Design review of the part built by this model. Coordinates are the model's own, in mm. Face numbers are marked on the shaded views. A direction names the side the tool comes from. Coordinates: 2 decimals unless noted, no trailing zeros. Order: outer loops, then holes, each group sorted by start corner. A loop starts at its lowest first (then second) coordinate and runs counter-clockwise, first axis right, second up. Notation, with made-up numbers: M -2,57 L 21,57 A12 cw 21,65 Z; hole C -18,23.5 d9. An arc over 180 degrees is marked long. Use CSV: the item, a comma, the result in double quotes.
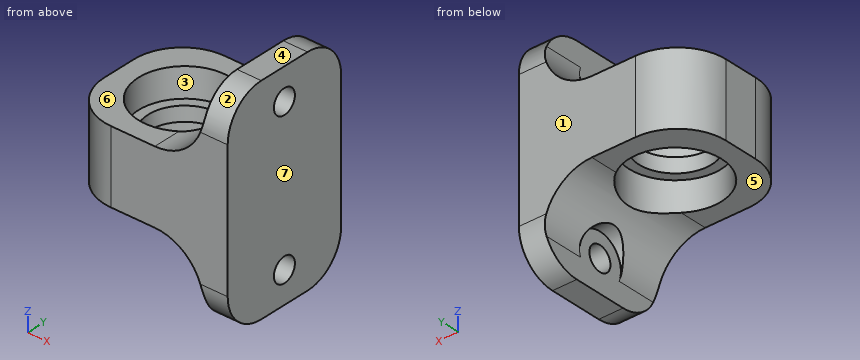
Autodesk Inventor part; units mm, degrees
ref_plane "YZ Plane" through (0, 0, 0) normal (1, 0, 0) x (0, 1, 0)
ref_plane "XZ Plane" through (0, 0, 0) normal (0, 1, 0) x (-1, 0, 0)
ref_plane "XY Plane" through (0, 0, 0) normal (0, 0, 1) x (1, 0, 0)
sketch "Szkic1" plane through (0, 0, 0) normal (0, 0, 1) x (1, 0, 0)
  line L0 (-15.5705, 13.388) -> (18.4295, 13.388)
  line L1 (18.4295, 13.388) -> (18.4295, -13.612)
  line L2 (18.4295, -13.612) -> (-15.5705, -13.612)
  line L3 (-15.5705, -13.612) -> (-15.5705, 13.388)
  circle A0 centre (-2.0705, -0.112) radius 9.5
  point P0 (0, 0)
  dimension "d0" = 27
  dimension "d1" = 34
  dimension "d2" = 20.5
  dimension "d3" = 13.5
  dimension "d4" = 19
extrude "Wyciągnięcie proste1" add sketch "Szkic1" along normal blind 15 contours L0 L1 L2 L3 | A0
extrude "Wyciągnięcie proste2" cut sketch "Szkic1" along normal blind 6 contours A0
sketch "Szkic2" plane through (0, 0, 15) normal (0, 0, 1) x (1, 0, 0)
  circle A0 centre (-2.0705, -0.112) radius 9.5
  line L0 (18.4295, 13.388) -> (-15.5705, 13.388)
  line L1 (-15.5705, 13.388) -> (-15.5705, -13.612)
  line L2 (-15.5705, -13.612) -> (18.4295, -13.612)
  line L3 (18.4295, -13.612) -> (18.4295, 13.388)
  point P0 (0, 0)
extrude "Wyciągnięcie proste3" cut sketch "Szkic2" against normal blind 6 contours A0
hole "Otwór1" at (-2.0705, -0.112, 0) direction (0, 0, 1) diameter 15 end through all
fillet "Zaokrąglenie1" radius 10 2 edges at (-15.5705, 13.388, 7.5) (-15.5705, -13.612, 7.5)
sketch "Szkic3" plane through (18.4295, -13.612, 0) normal (1, 0, 0) x (0, 0, -1)
  line L0 (0, 27) -> (0, 0)
  line L1 (0, 27) -> (-15, 27)
  line L2 (-15, 0) -> (-15, 27)
  line L3 (0, 0) -> (-15, 0)
  line L4 (-15, 27) -> (-29.5, 27)
  line L5 (-29.5, 27) -> (-29.5, 0)
  line L6 (-29.5, 0) -> (-15, 0)
  line L7 (0, 27) -> (14.5, 27)
  line L8 (14.5, 27) -> (14.5, 0)
  line L9 (14.5, 0) -> (0, 0)
  point P0 (0, 13.612)
  point P1 (-23, 13.5)
  point P2 (8, 13.5)
  dimension "d21" = 14.5
  dimension "d22" = 14.5
  dimension "d23" = 6.5
  dimension "d24" = 6.5
  dimension "d25" = 27
  dimension "d26" = 13.5
  dimension "d27" = 13.5
extrude "Wyciągnięcie proste4" add sketch "Szkic3" against normal blind 5 contours L7 L8 L9 L0 | L2 L6 L5 L4
hole "Otwór2" at (18.4295, -0.112, 23) at (18.4295, -0.112, -8) direction (-1, 0, 0) diameter 5 end through all
fillet "Zaokrąglenie2" radius 10 2 edges at (13.4295, -0.112, 15) (13.4295, -0.112, 0)
fillet "Zaokrąglenie3" radius 8 4 edges at (15.9295, 13.388, -14.5) (15.9295, -13.612, -14.5) (15.9295, -13.612, 29.5) (15.9295, 13.388, 29.5)
sketch "Szkic4" plane through (13.4295, -13.612, 0) normal (-1, 0, 0) x (0, 0, 1)
  arc A0 (-10, 15) -> (-10, 12) centre (-8, 13.5) ccw
  arc A1 (25, 12) -> (25, 15) centre (23, 13.5) ccw
  circle A2 centre (-8, 13.5) radius 5
  circle A3 centre (23, 13.5) radius 5
  point P0 (0, 13.612)
  dimension "d37" = 10
  dimension "d38" = 10
extrude "Wyciągnięcie proste5" cut sketch "Szkic4" along normal blind 5
properties part number "3DP_ABS_Y_Axis_Pulley_Rod_Mid_Bearing_Block"
(1) Add section B-B on x = 15. State the section outline as (y, z) points, and give its area (3 significant figures).
The answers:
outline,"M -13.61,-6.5 A8 ccw -5.61,-14.5 L 5.39,-14.5 A8 ccw 13.39,-6.5 L 13.39,21.5 A8 ccw 5.39,29.5 L -5.61,29.5 A8 ccw -13.61,21.5 Z; hole C -0.11,-8 d5; hole C -0.11,23 d5"
area,"1,090 mm2"
(2) For the marked faces 5, 6 and 7, list the 3-axis set-ups (+Z, -Z, +X, -X, +Y, -Y) from which the entire face can be reached by the end or side of a thin tool; tool diameter is ignored.
The answers:
face 5,"-Z, -X, +Y, -Y"
face 6,"+Z, -X, +Y, -Y"
face 7,"+Z, -Z, +X, +Y, -Y"
(3) Wall thickness on probe 1 along Z at (x, y) = (-7, 8.25); probe 2 along X at (y, z) = (5, 3.5); probe 3 along X at (y, z) = (12, 21): over which ranges is each line inside the solid? List them lowest first.
The answers:
probe 1,"z = 0 to 15"
probe 2,"x = -15.44 to -10.08, 5.94 to 18.43"
probe 3,"x = 12.59 to 18.43"
(4) Clearance check with flat-ended pins moving along their axes: P1, Ø5.5, axis at x = -3, y = -4, coming from the +Z side; P2, Ø8, axis at y = -0.112, z = 23, coming from the -X side; P3, Ø9.5, axis at x = -5, y = 2.5, coming from the -Z side; P4, Ø5, axis at x = 7.5, y = 0.5, coming from the -Z side. State where each tip first meets the part, or that it passes through.
The answers:
P1,"passes through"
P2,"stops at x = 13.43"
P3,"stops at z = 6"
P4,"stops at z = -2.46"
(5) Add section A-A on z = 7. State the section outline as (x, y) points, and give its area (3 significant figures).
The answers:
outline,"M -15.57,-3.61 A10 ccw -5.57,-13.61 L 18.43,-13.61 L 18.43,13.39 L -5.57,13.39 A10 ccw -15.57,3.39 Z; hole C -2.07,-0.11 d15"
area,"698 mm2"
(6) The part is to be moulded in two halves that separate along Y. For the marked faces 1, 2, 3 and 4, say which applies: pulls with the +Y half, pulls with the -Y half, needs draft (parallel to the pull), parting line crosses it, or undercut.
The answers:
face 1,"pulls with the +Y half"
face 2,"pulls with the -Y half"
face 3,"undercut"
face 4,"needs draft"
(7) Add section D-D on y = 10.5. State the section outline as (x, z) points.
The answers:
outline,"M -12.6,0 L 3.43,0 A10 cw 13.43,-10 L 13.43,-12.65 L 18.43,-12.65 L 18.43,27.65 L 13.43,27.65 L 13.43,25 A10 cw 3.43,15 L -12.6,15 Z"
(8) Add section C-C on z = 23. State the section outline as (x, y) points.
The answers:
outline,"M 13.23,-13.47 L 18.43,-13.47 L 18.43,-2.61 L 13.43,-2.61 L 13.43,-5.11 L 13.23,-5.11 Z; M 13.23,4.89 L 13.43,4.89 L 13.43,2.39 L 18.43,2.39 L 18.43,13.25 L 13.23,13.25 Z"
